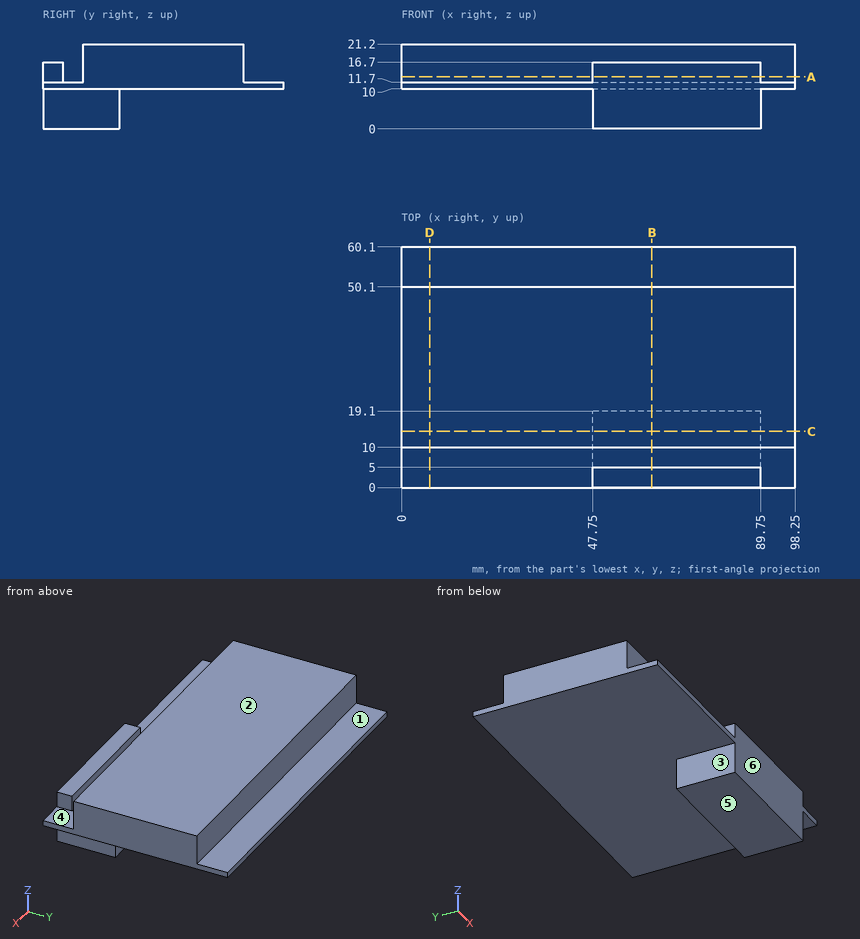
Design review of the part shown in the three views and the two pictorial views. Dimensions are in mm from the part's minimum x, y and z. A direction names the side the tool comes from. Coordinates: 2 decimals unless noted, no trailing zeros. Order: outer loops, then holes, each group sorted by start corner. A loop starts at its lowest first (then second) coordinate and runs counter-clockwise, first axis right, second up.
1) Take a section at C-C, the plane y = 14. Give the boundary of the cut face in (x, z), and give its area (3 significant figures).
2) Clearance check with flat-ended pins moving along their axes: pin 1 (8 mm diameter, centred on x = 52.5, y = 56.5, fed in from +Z); pin 2 (1.5 mm diameter, centred on y = 2, z = 15.5, fed in from +X); pin 3 (1.5 mm diameter, centred on y = 16, z = 4.5, fed in from -X). State where each tip first meets the part, or that it passes through.
3) Take a section at B-B, the plane x = 62.5. Give the boundary of the cut face in (y, z).
4) Wall thickness on line 1 along Y through (x, z) = (59, 12.75); line 2 along Z through (x, y) = (37, 8.5); line 3 along Y through (x, z) = (77.5, 2.5): over which ranges is each line inside the solid? List them lowest first.
5) For the marked faces 1, 2 and 3, list the 3-axis set-ups (+Z, -Z, +X, -X, +Y, -Y) from which the entire face can be reached by the end or side of a thin tool; tool diameter is ignored.
6) Take a section at D-D, the plane x = 7. Give the boundary of the cut face in (y, z), and give its area (3 significant figures).
7) Mouldability with a two-part tool opening along Y and no side actions: class the marked faces 4, 5 and 6 as +Y half, -Y half, draft (parallel to the pull), parting line (faces both ways), or undercut.
8) Take a section at A-A, the plane z = 13. Give the boundary of the cut face in (x, y).
Returned:
1. outline: (0, 10) - (47.75, 10) - (47.75, 0) - (89.75, 0) - (89.75, 10) - (98.25, 10) - (98.25, 21.2) - (0, 21.2) - close
1. area: 1,520 mm2
2. pin 1: stops at z = 11.7
2. pin 2: stops at x = 89.75
2. pin 3: stops at x = 47.75
3. outline: (0, 0) - (19.1, 0) - (19.1, 10) - (60.1, 10) - (60.1, 11.7) - (50.1, 11.7) - (50.1, 21.2) - (10, 21.2) - (10, 11.7) - (5, 11.7) - (5, 16.7) - (0, 16.7) - close
4. line 1: y = 0 to 5, 10 to 50.1
4. line 2: z = 10 to 11.7
4. line 3: y = 0 to 19.1
5. face 1: +Z, +X, -X, +Y
5. face 2: +Z, +X, -X, +Y, -Y
5. face 3: -Z, -X, +Y, -Y
6. outline: (0, 10) - (60.1, 10) - (60.1, 11.7) - (50.1, 11.7) - (50.1, 21.2) - (10, 21.2) - (10, 11.7) - (0, 11.7) - close
6. area: 483 mm2
7. face 4: undercut
7. face 5: draft
7. face 6: -Y half
8. outline: (0, 10) - (98.25, 10) - (98.25, 50.1) - (0, 50.1) - close; (47.75, 0) - (89.75, 0) - (89.75, 5) - (47.75, 5) - close
